```python
from build123d import *

# Parameters (mm, degrees)
F1_DEPTH = 4
F2_R     = 4
F3_R     = 1.99999
F4_R     = 3
F5_R     = 7


# Not quite as in the source:
# - a fillet or chamfer is up to 0.001 mm smaller than in the source, because OpenCascade refuses the exact size


with BuildPart() as f1:
    # F0 (on Front) → F1 (new body)
    with BuildSketch(Plane.XZ):
        Polygon((9, 4.5), (9, 12.5), (-6, 12.5), (-6, -12.5), (6, -12.5), (6, -4.5), (2, -4.5), (2, -8.5), (-2, -8.5), (-2, 8.5), (5, 8.5), (5, 4.5), align=None)
    extrude(amount=F1_DEPTH)

    # F2
    f2_edges = [f1.edges().sort_by_distance(p)[0] for p in [
        (9, -2, 12.5),
        (-6, -2, -12.5),
        (6, -2, -12.5),
    ]]
    fillet(f2_edges, radius=F2_R)

    # F3 (radius 2 in the source; OpenCascade refuses exactly that, so slightly less here)
    f3_edges = [f1.edges().sort_by_distance(p)[0] for p in [
        (6, -2, -4.5),
        (2, -2, -4.5),
        (9, -2, 4.5),
        (5, -2, 4.5),
    ]]
    fillet(f3_edges, radius=F3_R)

    # F4
    f4_edges = [f1.edges().sort_by_distance(p)[0] for p in [
        (-2, -2, 8.5),
    ]]
    fillet(f4_edges, radius=F4_R)

    # F5
    f5_edges = [f1.edges().sort_by_distance(p)[0] for p in [
        (-6, -2, 12.5),
    ]]
    fillet(f5_edges, radius=F5_R)


solid = f1.part
```
Input: part model. Units: mm. Frame: model coordinates. A direction names the side the tool comes from. Round coordinates to 2 decimals unless told otherwise and drop trailing zeros. Order: outer loops, then holes, each group sorted by start corner. A loop starts at its lowest first (then second) coordinate and runs counter-clockwise, first axis right, second up. Notation, with made-up numbers: (88.25, -17) - (124.25, -17) arc R22 ccw to (124.25, 19) - close; hole circle Ø3 at (9.25, 32.25). An arc over 180 degrees is marked (long way). Answer in a Markdown table with one row per item.
Item 1: Mould query, pull axis Z, two halves, no side actions, for faces 1 (the flat face through (-4, 0, 0)), 2 (the cylindrical face through (5.43, -2.03, -5.1)), 3 (the cylindrical face through (4.797, -2.028, -11.359)), 4 (the cylindrical face through (7.859, -2.028, 11.297)). Classes: released by +Z, released by -Z, zero draft, split by the parting line, or undercut.
Model answer:
| item | result |
|---|---|
| face 1 | zero draft |
| face 2 | undercut |
| face 3 | released by -Z |
| face 4 | released by +Z |
Item 2: Pin query (flat end, axial travel): pin 1 (2 mm diameter, centred on y = -1.5, z = 0.5, fed in from +X); pin 2 (2 mm diameter, centred on y = -3.5, z = 7.5, fed in from -X); pin 3 (1.5 mm diameter, centred on x = -2.5, y = -2.5, fed in from +Z). Return the tip coordinate at first contact, or that it passes through.
Model answer:
| item | result |
|---|---|
| pin 1 | stops at x = -2 |
| pin 2 | stops at x = -5.93 |
| pin 3 | stops at z = 11.94 |
Item 3: Reachability of faces 5 (the cylindrical face through (2.57, -2.03, -5.1)), 6 (the flat face through (-6, -2, -1)) from +Z, -Z, +X, -X, +Y, -Y: full face, straight path, thin tool, end or side. Return the list, or none.
Model answer:
| item | result |
|---|---|
| face 5 | +Y, -Y |
| face 6 | +Z, -Z, -X, +Y, -Y |
Item 4: Section query D-D (z = 4.25). Return the cut outline in (x, y).
Model answer:
| item | result |
|---|---|
| outline | (-6, -4) - (-2, -4) - (-2, 0) - (-6, 0) - close |
Item 5: Section query B-B (z = -8.25). Return the cut outline in (x, y), then the cut area to 3 significant figures.
Model answer:
| item | result |
|---|---|
| outline | (-6, -4) - (-2, -4) - (-2, 0) - (-6, 0) - close; (2, -4) - (6, -4) - (6, 0) - (2, 0) - close |
| area | 32.0 mm² |
Item 6: Section query A-A (x = 1.75). Return the cut outline in (y, z), then the cut area to 3 significant figures.
Model answer:
| item | result |
|---|---|
| outline | (-4, -12.5) - (0, -12.5) - (0, -8.5) - (-4, -8.5) - close; (-4, 8.5) - (0, 8.5) - (0, 12.5) - (-4, 12.5) - close |
| area | 32.0 mm² |
Item 7: Line query: line 1 (X direction, y = -2.45, z = -6.5); line 2 (Z direction, x = 1.75, y = -1.85); line 3 (X direction, y = -2.9, z = 0.75). Output: solid intervals per line, ascending.
Model answer:
| item | result |
|---|---|
| line 1 | x = -6 to -2, 2 to 6 |
| line 2 | z = -12.5 to -8.5, 8.5 to 12.5 |
| line 3 | x = -6 to -2 |
